Design review of the part shown in the three views and the two pictorial views. Dimensions are in mm from the part's minimum x, y and z. Coordinates: 2 decimals unless noted, no trailing zeros. Loops run counter-clockwise (first coordinate to the right, second up) from the corner with the lowest first, then second, coordinate; pieces in that order, holes last. Notation, with made-up numbers: (46, 83.25) - (50, 83.25) arc R21 cw to (50, 114.25) - close; hole circle Ø8 at (4, 61.5). An arc over 180 degrees is marked (long way). One line per item, written item: value. Start each with the question number.
1. To check wall thickness, follow line 1 (X direction, y = 5.5, z = 6.5); line 2 (Z direction, x = 6, y = 7.25); line 3 (Y direction, x = 20, z = 19.5). State the ranges of each line that lie inside material, in increasing order. Write a range as from..to.
2. Insertion check: pin 1 (3 mm diameter, centred on y = 3, z = 28.5, fed in from +X); pin 2 (4 mm diameter, centred on x = 29.5, y = 2, fed in from +Z); pin 3 (5 mm diameter, centred on x = 12, z = 28, fed in from -Y). Each pin has a flat end and moves straight along its axis. Give the tip position at first contact, or say it passes through.
3. Take a section at C-C, the plane x = 47. State the section outline as (y, z) points.
4. Take a section at A-A, the plane x = 36. State the section outline as (y, z) points, and give its area (3 significant figures).
5. Take a section at D-D, the plane z = 15. State the section outline as (x, y) points, and give its area (3 significant figures).
6. The part is to be moulded in two halves that separate along Z. For the marked faces 1 and 2, say which applies: released by +Z, released by -Z, zero draft, split by the parting line, or undercut.
7. Take a section at B-B, the plane z = 6. State the section outline as (x, y) points.
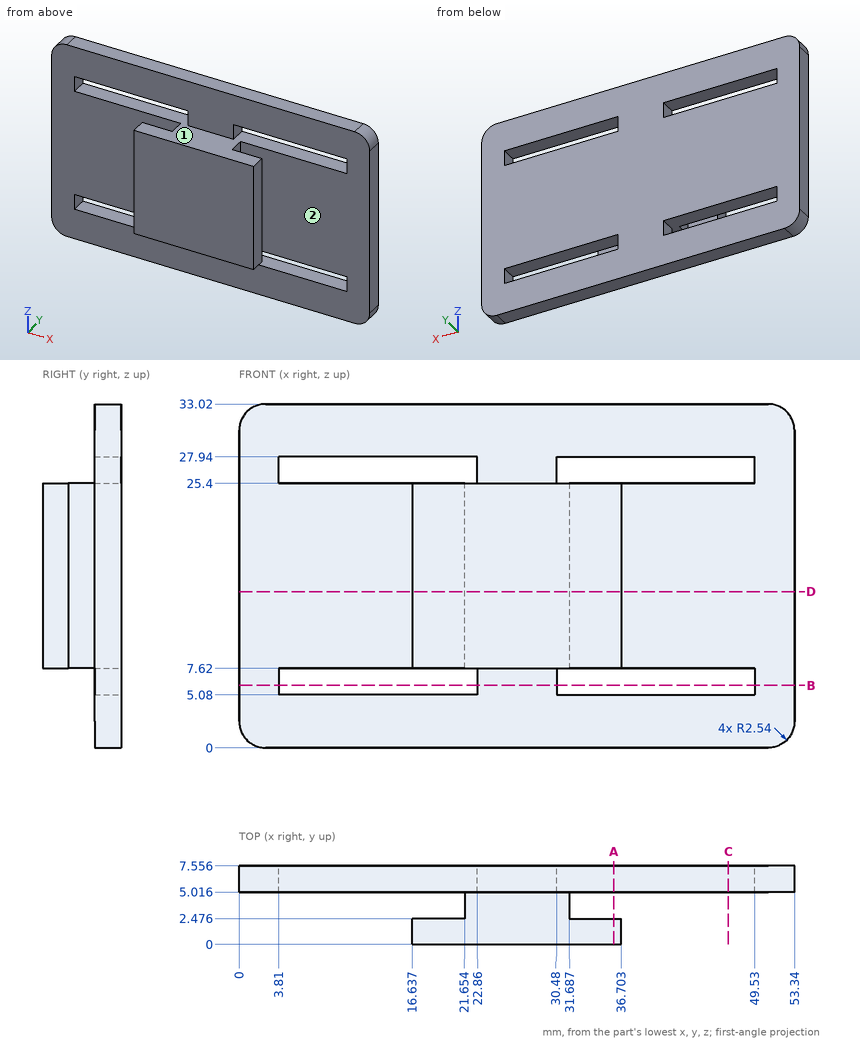
Solutions:
1. line 1: 0..3.81, 22.86..30.48, 49.53..53.34
1. line 2: 0..5.08, 7.62..25.4, 27.94..33.02
1. line 3: 0..2.48, 5.02..7.56
2. pin 1: through
2. pin 2: z = 25.4
2. pin 3: y = 5.02
3. outline: (5.02, 0) - (7.56, 0) - (7.56, 5.08) - (5.02, 5.08) - close; (5.02, 7.62) - (7.56, 7.62) - (7.56, 25.4) - (5.02, 25.4) - close; (5.02, 27.94) - (7.56, 27.94) - (7.56, 33.02) - (5.02, 33.02) - close
4. outline: (0, 7.62) - (2.48, 7.62) - (2.48, 25.4) - (0, 25.4) - close; (5.02, 0) - (7.56, 0) - (7.56, 5.08) - (5.02, 5.08) - close; (5.02, 7.62) - (7.56, 7.62) - (7.56, 25.4) - (5.02, 25.4) - close; (5.02, 27.94) - (7.56, 27.94) - (7.56, 33.02) - (5.02, 33.02) - close
4. area: 115 mm2
5. outline: (0, 5.02) - (21.65, 5.02) - (21.65, 2.48) - (16.64, 2.48) - (16.64, 0) - (36.7, 0) - (36.7, 2.48) - (31.69, 2.48) - (31.69, 5.02) - (53.34, 5.02) - (53.34, 7.56) - (0, 7.56) - close
5. area: 211 mm2
6. face 1: undercut
6. face 2: zero draft
7. outline: (0, 5.02) - (3.81, 5.02) - (3.81, 7.56) - (0, 7.56) - close; (22.86, 5.02) - (30.48, 5.02) - (30.48, 7.56) - (22.86, 7.56) - close; (49.53, 5.02) - (53.34, 5.02) - (53.34, 7.56) - (49.53, 7.56) - close
